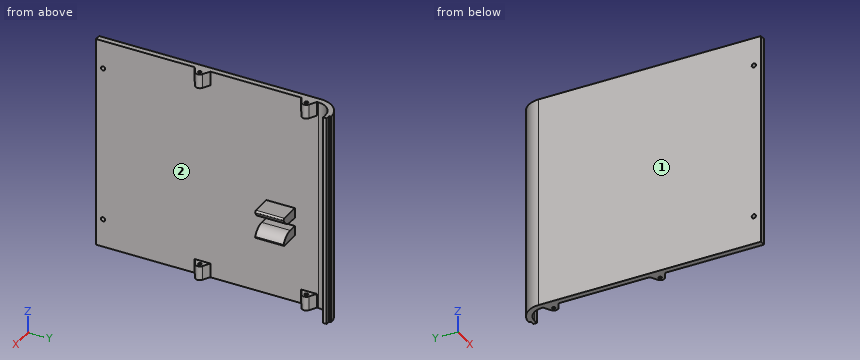
```python
from build123d import *

# Parameters (mm, degrees)
EXTRU_MINCE1_DEPTH                   = 75
ESQUISSE2_R                          = 1.5
ENL_V_MAT_EXTRU_1_DEPTH              = 188.782453919
ESQUISSE3_W                          = 3
ESQUISSE3_H                          = 2.5
BOSS_EXTRU_1_DEPTH                   = 150
ESQUISSE4_R                          = 1.2
BOSS_EXTRU_2_DEPTH                   = 10
R_P_TITION_LIN_AIRE1_COUNT           = 2
R_P_TITION_LIN_AIRE1_PITCH           = 75
R_P_TITION_LIN_AIRE1_COPY_1_SKETCH_R = 1.2
R_P_TITION_LIN_AIRE1_COPY_1_DEPTH    = 10
BOSS_EXTRU_3_START                   = -120
BOSS_EXTRU_3_DEPTH                   = 20
CONG_1_R                             = 1


with BuildPart() as part:
    # Esquisse1 → Extru.-Mince1 (new, symmetric)
    with BuildSketch(Plane.XY):
        with BuildLine():
            Line((0, 0), (0, 156.5))
            ThreePointArc((0, 156.5), (4.393398282, 167.106601718), (15, 171.5))
            Line((15, 171.5), (15, 167.5))
            ThreePointArc((15, 167.5), (7.221825407, 164.278174593), (4, 156.5))
            Line((4, 156.5), (4, 0))
            Line((4, 0), (0, 0))
        make_face()
    extrude(amount=EXTRU_MINCE1_DEPTH, both=True)

    # Esquisse2 → Enlèv. mat.-Extru.1 (cut, through all)
    with BuildSketch(Plane.ZY):
        with Locations((-55, 5)):
            Circle(ESQUISSE2_R)
        with Locations((55, 5)):
            Circle(ESQUISSE2_R)
    extrude(amount=-ENL_V_MAT_EXTRU_1_DEPTH, mode=Mode.SUBTRACT)

    # Esquisse3 → Boss.-Extru.1 (add)
    with BuildSketch(Plane.XY.offset(75)):
        with Locations((16.5, 168.75)):
            Rectangle(ESQUISSE3_W, ESQUISSE3_H)
    extrude(amount=-BOSS_EXTRU_1_DEPTH)

    # Esquisse4 → Boss.-Extru.2 (add)
    with BuildSketch(Plane.XY.offset(75)):
        with BuildLine():
            Line((4, 155.484827557), (9, 152.598076211))
            ThreePointArc((9, 152.598076211), (10.5, 150), (9, 147.401923789))
            Line((9, 147.401923789), (4, 144.515172443))
            Line((4, 144.515172443), (4, 155.484827557))
        make_face()
        with Locations((7.5, 150)):
            Circle(ESQUISSE4_R, mode=Mode.SUBTRACT)
    boss_extru_2 = extrude(amount=-BOSS_EXTRU_2_DEPTH)

    # Symétrie1: Boss.-Extru.2 across plane
    add(boss_extru_2.mirror(Plane.XY))

    # Répétition linéaire1: Boss.-Extru.2 ×2
    with Locations(*[(0, -i * R_P_TITION_LIN_AIRE1_PITCH, 0) for i in range(1, R_P_TITION_LIN_AIRE1_COUNT)]):
        add(boss_extru_2)

    # Répétition linéaire1 copy 1 sketch → Répétition linéaire1 copy 1 (add)
    with BuildSketch(Plane(origin=(0, -75, -75), x_dir=(1, 0, 0), z_dir=(0, 0, -1))):
        with BuildLine():
            Line((4, -155.484827557), (9, -152.598076211))
            ThreePointArc((9, -152.598076211), (10.5, -150), (9, -147.401923789))
            Line((9, -147.401923789), (4, -144.515172443))
            Line((4, -144.515172443), (4, -155.484827557))
        make_face()
        with Locations((7.5, -150)):
            Circle(R_P_TITION_LIN_AIRE1_COPY_1_SKETCH_R, mode=Mode.SUBTRACT)
    extrude(amount=-R_P_TITION_LIN_AIRE1_COPY_1_DEPTH)

    # Esquisse5 → Boss.-Extru.3 (add)
    with BuildSketch(Plane.XZ.offset(BOSS_EXTRU_3_START)):
        with BuildLine():
            Line((4, -14), (10, -14))
            ThreePointArc((10, -14), (15.700877125, -12.043984876), (19, -7))
            Line((19, -7), (4, -7))
            Line((4, -7), (4, -14))
        make_face()
        with BuildLine():
            Line((4, -27), (4, -20))
            Line((4, -20), (10, -20))
            ThreePointArc((10, -20), (15.700877125, -21.956015124), (19, -27))
            Line((19, -27), (4, -27))
        make_face()
    extrude(amount=-BOSS_EXTRU_3_DEPTH)

    # Congé1
    cong_1_edges = [part.edges().sort_by_distance(p)[0] for p in [
        (19, 130, -7),
        (19, 130, -27),
    ]]
    fillet(cong_1_edges, radius=CONG_1_R)


solid = part.part
```
Part model, mm, in its own coordinate system. Face numbers are marked on the shaded views. Round coordinates to 2 decimals unless told otherwise and drop trailing zeros. Order: outer loops, then holes, each group sorted by start corner. A loop starts at its lowest first (then second) coordinate and runs counter-clockwise, first axis right, second up. Notation, with made-up numbers: M 50,34 L 80,34 A12 ccw 80,49 Z; hole C -3,17.5 d5. An arc over 180 degrees is marked long. Put each result on its own line as item: value. Start each with the question number.
1. Drill centre lines: probe 1 along X at (y, z) = (75, 71); probe 2 along Y at (x, z) = (7.5, -72); probe 3 along X at (y, z) = (122, -49.5). Where is each one in solid material? Low to high. Write a range as [from, to].
2. Slice it at A-A on z = 9. List the corners of the cut face in (x, y), then the cut area to 3 significant figures.
3. Two-plate mould, pull along Z, no slides. Class the marked faces 1 and 2: +Z half, -Z half, draft (parallel to the pull), parting line (faces both ways), or undercut.
4. Drop flat-ended pins along their axis: pin 1 (1 mm diameter, centred on x = 8.5, z = -14, fed in from -Y); pin 2 (3.5 mm diameter, centred on y = 5, z = 55, fed in from +X); pin 3 (1.5 mm diameter, centred on x = 11, z = 9.5, fed in from +Y); pin 4 (1.8 mm diameter, centred on y = 5, z = -55, fed in from +X). Give the stop position or say it passes through.
5. Slice it at B-B on y = 88.5. List the corners of the cut face in (x, z), then the cut area to 3 significant figures.
Findings:
1. probe 1: [0, 6.3], [8.7, 10.5]
1. probe 2: [71.54, 73.8], [76.2, 78.46], [146.54, 148.8], [151.2, 153.46], [164.55, 169.49]
1. probe 3: [0, 4]
2. outline: M 0,0 L 4,0 L 4,156.5 A11 cw 15,167.5 L 18,167.5 L 18,170 L 15,170 L 15,171.5 A15 ccw 0,156.5 Z
2. area: 715 mm2
3. face 1: draft
3. face 2: undercut
4. pin 1: y = 120
4. pin 2: x = 4
4. pin 3: y = 171.14
4. pin 4: through
5. outline: M 0,-75 L 4,-75 L 4,75 L 0,75 Z
5. area: 600 mm2
